```python
from build123d import *

# Parameters (mm, degrees)
SKETCH1_R           = 1.5
BOSS_EXTRUDE1_DEPTH = 50
SKETCH2_R           = 5.5
BOSS_EXTRUDE2_DEPTH = 10
FILLET1_R           = 1


with BuildPart() as part:
    # Sketch1 → Boss-Extrude1 (new body)
    with BuildSketch(Plane.XY):
        with Locations((0, 12.02081528)):
            Circle(SKETCH1_R)
    extrude(amount=BOSS_EXTRUDE1_DEPTH)

    # Sketch2 → Boss-Extrude2 (add)
    with BuildSketch(Plane.XY.offset(50)):
        with Locations((0, 12.02081528)):
            Circle(SKETCH2_R)
    extrude(amount=BOSS_EXTRUDE2_DEPTH)

    # Fillet1
    fillet1_edges = [part.edges().sort_by_distance(p)[0] for p in [
        (-5.5, 12.02081528, 50),
        (-5.5, 12.02081528, 60),
    ]]
    fillet(fillet1_edges, radius=FILLET1_R)


solid = part.part
```
The model under review builds one solid part; all positions refer to its coordinate system, in mm. A direction names the side the tool comes from. Round coordinates to 2 decimals unless told otherwise and drop trailing zeros. Loops run counter-clockwise (first coordinate to the right, second up) from the corner with the lowest first, then second, coordinate; pieces in that order, holes last. Notation, with made-up numbers: M 73.25,34 L 100.25,34 A18 ccw 100.25,57 Z; hole C -38.75,48.5 d1. An arc over 180 degrees is marked long. Write item = value, one per line.
Item 1: Take a section at A-A on x = 0. Write out the cut boundary in (y, z).
Return value:
outline = M 6.52,51 A1 ccw 7.52,50 L 10.52,50 L 10.52,0 L 13.52,0 L 13.52,50 L 16.52,50 A1 ccw 17.52,51 L 17.52,59 A1 ccw 16.52,60 L 7.52,60 A1 ccw 6.52,59 Z
Item 2: For line 1 (Z direction, x = -0.25, y = 16.5); line 2 (X direction, y = 11.5, z = 7.5); line 3 (Z direction, x = 4.75, y = 13.5), list the stretches that pass through material, from the lowest coordinate up. Write a range as [from, to].
Return value:
line_1 = [50, 60]
line_2 = [-1.41, 1.41]
line_3 = [50.12, 59.88]
Item 3: Insertion check: P1, Ø1, axis at x = 3.5, z = 52, coming from the +Y side; P2, Ø3, axis at y = 12.5, z = 46.5, coming from the -X side; P3, Ø2, axis at x = -2.5, y = 9.5, coming from the -Z side. Each pin has a flat end and moves straight along its axis. Give the tip position at first contact, or say it passes through.
Return value:
P1 = 16.63
P2 = -1.5
P3 = 50
Item 4: Machinability: for faces 1 (the flat face through (0, 12, 60)), 2 (the cylindrical face through (-0.325, 10.556, 24.65)), which of the approach directions +Z, -Z, +X, -X, +Y, -Y give a long, thin tool a straight path to every point of the face, cutting with its end or side? Answer none if there is none.
Return value:
face_1 = +Z, +X, -X, +Y, -Y
face_2 = -Z
Item 5: Take a section at B-B on z = 21. Write out the cut boundary in (x, y).
Return value:
outline = C 0,12.02 d3
